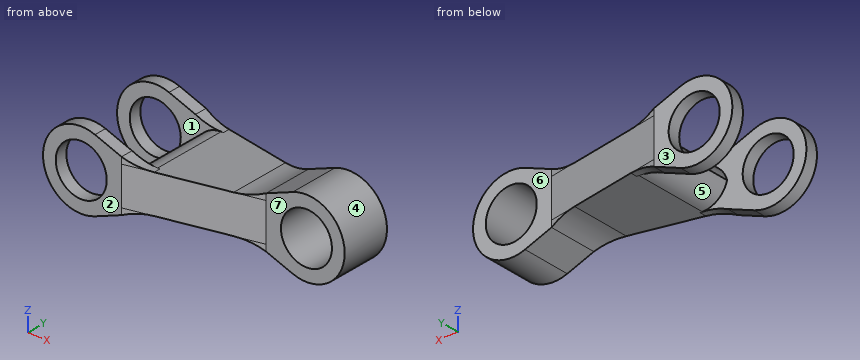
from build123d import *

# Parameters (mm, degrees)
SKETCH1_R           = 5.08
BOSS_EXTRUDE1_DEPTH = 10.16
SKETCH2_W           = 15.638324702
SKETCH2_H           = 15.24
CUT_EXTRUDE1_DEPTH  = 54.836616721
FILLET1_R           = 12.7
FILLET2_R           = 5.08


with BuildPart() as part:
    # Sketch1 → Boss-Extrude1 (new, symmetric)
    with BuildSketch(Plane(origin=(0, 0, 0), x_dir=(1, 0, 0), z_dir=(0, 1, 0))):
        with BuildLine():
            Line((2.735663722, 7.112), (8.018324702, 5.08))
            Line((8.018324702, 5.08), (8.018324702, 3.81))
            Line((8.018324702, 3.81), (32.621675298, 3.81))
            Line((32.621675298, 3.81), (32.621675298, 5.08))
            Line((32.621675298, 5.08), (37.904336278, 7.112))
            ThreePointArc((37.904336278, 7.112), (48.26, 0), (37.904336278, -7.112))
            Line((37.904336278, -7.112), (32.621675298, -5.08))
            Line((32.621675298, -5.08), (32.621675298, -3.81))
            Line((32.621675298, -3.81), (8.018324702, -3.81))
            Line((8.018324702, -3.81), (8.018324702, -5.08))
            Line((8.018324702, -5.08), (2.735663722, -7.112))
            ThreePointArc((2.735663722, -7.112), (-7.62, 0), (2.735663722, 7.112))
        make_face()
        with Locations(Location((0, 0, 0), (0, 0, 270))):
            Circle(SKETCH1_R, mode=Mode.SUBTRACT)
        with Locations(Location((40.64, 0, 0), (0, 0, 270))):
            Circle(SKETCH1_R, mode=Mode.SUBTRACT)
    extrude(amount=BOSS_EXTRUDE1_DEPTH, both=True)

    # Sketch2 → Cut-Extrude1 (cut, through all)
    with BuildSketch(Plane.XY.offset(13.97)):
        Polygon((8.018324702, 10.16), (32.621675298, 5.08), (48.26, 5.08), (48.26, 10.16), align=None)
        with Locations((0.199162351, 0)):
            Rectangle(SKETCH2_W, SKETCH2_H)
        Polygon((48.26, -10.16), (48.26, -5.08), (32.621675298, -5.08), (8.018324702, -10.16), align=None)
    extrude(amount=-CUT_EXTRUDE1_DEPTH, mode=Mode.SUBTRACT)

    # Fillet1
    # the kernel refuses this fillet: 12.7 mm, written as the material it adds along each edge
    with BuildSketch(Plane(origin=(32.621675298, 18.919504146, 3.81), x_dir=(-1, 0, 0), z_dir=(0, -1, 0))) as fillet1_piece_1_section:
        with BuildLine():
            CenterArc((5.535801658, -12.7), FILLET1_R, 90, 25.841932763)
            Line((0, -1.27), (0, 0))
            Line((0, 0), (5.535801658, 0))
        make_face()
    fillet1_piece_1 = extrude(amount=37.839008291, mode=Mode.PRIVATE)
    fillet1_piece_1 = split(fillet1_piece_1, bisect_by=Plane(origin=(37.374376864, -4.098681465, 3.81), z_dir=(-0.20221057606968723, 0.9793420663514691, 0)), keep=Keep.TOP, mode=Mode.PRIVATE)
    fillet1_piece_1 = split(fillet1_piece_1, bisect_by=Plane(origin=(29.880992297, 5.645885105, 3.81), z_dir=(-0.20221057606968723, -0.9793420663514691, 0)), keep=Keep.TOP, mode=Mode.PRIVATE)
    add(fillet1_piece_1)
    with BuildSketch(Plane(origin=(32.621675298, 18.919504146, -3.81), x_dir=(-1, 0, 0), z_dir=(0, -1, 0))) as fillet1_piece_2_section:
        with BuildLine():
            CenterArc((5.535801658, 12.7), FILLET1_R, 244.158067237, 25.841932763)
            Line((0, 1.27), (0, 0))
            Line((0, 0), (5.535801658, 0))
        make_face()
    fillet1_piece_2 = extrude(amount=37.839008291, mode=Mode.PRIVATE)
    fillet1_piece_2 = split(fillet1_piece_2, bisect_by=Plane(origin=(37.374376864, -4.098681465, -3.81), z_dir=(-0.20221057606968723, 0.9793420663514691, 0)), keep=Keep.TOP, mode=Mode.PRIVATE)
    fillet1_piece_2 = split(fillet1_piece_2, bisect_by=Plane(origin=(29.880992297, 5.645885105, -3.81), z_dir=(-0.20221057606968723, -0.9793420663514691, 0)), keep=Keep.TOP, mode=Mode.PRIVATE)
    add(fillet1_piece_2)
    with BuildSketch(Plane(origin=(8.018324702, -7.62, -3.81), x_dir=(1, 0, 0), z_dir=(0, -1, 0))) as fillet1_piece_3_section:
        with BuildLine():
            CenterArc((5.535801658, -12.7), FILLET1_R, 90, 25.841932763)
            Line((0, -1.27), (0, 0))
            Line((0, 0), (5.535801658, 0))
        make_face()
    fillet1_piece_3 = extrude(amount=16.379504146, mode=Mode.PRIVATE)
    fillet1_piece_3 = split(fillet1_piece_3, bisect_by=Plane(origin=(8.521329344, -10.056141643, -3.81), z_dir=(-0.20221057606968723, 0.9793420663514691, 0)), keep=Keep.TOP, mode=Mode.PRIVATE)
    add(fillet1_piece_3)
    with BuildSketch(Plane(origin=(8.018324702, 23.999504146, -3.81), x_dir=(1, 0, 0), z_dir=(0, -1, 0))) as fillet1_piece_4_section:
        with BuildLine():
            CenterArc((5.535801658, -12.7), FILLET1_R, 90, 25.841932763)
            Line((0, -1.27), (0, 0))
            Line((0, 0), (5.535801658, 0))
        make_face()
    fillet1_piece_4 = extrude(amount=16.379504146, mode=Mode.PRIVATE)
    fillet1_piece_4 = split(fillet1_piece_4, bisect_by=Plane(origin=(5.277641702, 10.725885105, -3.81), z_dir=(-0.20221057606968723, -0.9793420663514691, 0)), keep=Keep.TOP, mode=Mode.PRIVATE)
    add(fillet1_piece_4)
    with BuildSketch(Plane(origin=(8.018324702, -7.62, 3.81), x_dir=(0, 0, 1), z_dir=(0, -1, 0))) as fillet1_piece_5_section:
        with BuildLine():
            CenterArc((12.7, -5.535801658), FILLET1_R, 154.158067237, 25.841932763)
            Line((0, -5.535801658), (0, 0))
            Line((0, 0), (1.27, 0))
        make_face()
    fillet1_piece_5 = extrude(amount=16.379504146, mode=Mode.PRIVATE)
    fillet1_piece_5 = split(fillet1_piece_5, bisect_by=Plane(origin=(8.521329344, -10.056141643, 3.81), z_dir=(-0.20221057606968723, 0.9793420663514691, 0)), keep=Keep.TOP, mode=Mode.PRIVATE)
    add(fillet1_piece_5)
    with BuildSketch(Plane(origin=(8.018324702, 23.999504146, 3.81), x_dir=(0, 0, 1), z_dir=(0, -1, 0))) as fillet1_piece_6_section:
        with BuildLine():
            CenterArc((12.7, -5.535801658), FILLET1_R, 154.158067237, 25.841932763)
            Line((0, -5.535801658), (0, 0))
            Line((0, 0), (1.27, 0))
        make_face()
    fillet1_piece_6 = extrude(amount=16.379504146, mode=Mode.PRIVATE)
    fillet1_piece_6 = split(fillet1_piece_6, bisect_by=Plane(origin=(5.277641702, 10.725885105, 3.81), z_dir=(-0.20221057606968723, -0.9793420663514691, 0)), keep=Keep.TOP, mode=Mode.PRIVATE)
    add(fillet1_piece_6)

    # Fillet2
    # the kernel refuses this fillet: 5.08 mm, written as the material it takes off along each edge
    with BuildSketch(Plane(origin=(8.018324702, 7.62, -3.81), x_dir=(1, 0, 0), z_dir=(0, -1, 0)), Plane(origin=(8.018324702, 7.62, 3.81), x_dir=(0, 0, -1), z_dir=(0, -1, 0))) as fillet2_piece_1:
        with BuildLine():
            CenterArc((FILLET2_R, FILLET2_R), FILLET2_R, 180, 90)
            Line((0, FILLET2_R), (0, 0))
            Line((0, 0), (FILLET2_R, 0))
        make_face()
    extrude(amount=15.24, mode=Mode.SUBTRACT)


solid = part.part
Read the model definition and answer for the solid it produces. Units are mm, in the model's axes. Face numbers are marked on the shaded views. A direction names the side the tool comes from. Round coordinates to 2 decimals unless told otherwise and drop trailing zeros. Write each loop counter-clockwise with the first axis right and the second up, starting at its lowest first coordinate (ties: lowest second). Pieces come first, ordered by that corner, then holes. Notation, with made-up numbers: M -1.5,38.25 L 31.5,38.25 A24 ccw 31.5,51.25 Z; hole C -20,-7.5 d11. An arc over 180 degrees is marked long. Use a Markdown table: item, result.
1) For a pull along Y with two mould halves and no side action, classify the marked faces 1, 2, 3 and 4 as pulls with the +Y half, pulls with the -Y half, needs draft (parallel to the pull), parting line crosses it, or undercut.
Answers follow:
| item | result |
|---|---|
| face 1 | undercut |
| face 2 | pulls with the -Y half |
| face 3 | pulls with the +Y half |
| face 4 | needs draft |
2) The part is cut by section C-C (z = 1.75). Write down the section's boundary in (x, y), plus the area to 3 significant figures.
Answers follow:
| item | result |
|---|---|
| outline | M -7.42,-10.16 L -4.77,-10.16 L -4.77,-7.62 L -7.42,-7.62 Z; M -7.42,7.62 L -4.77,7.62 L -4.77,10.16 L -7.42,10.16 Z; M 4.77,-10.16 L 8.02,-10.16 L 32.62,-5.08 L 35.87,-5.08 L 35.87,5.08 L 32.62,5.08 L 8.02,10.16 L 4.77,10.16 L 4.77,7.62 L 9.01,7.62 L 9.01,-7.62 L 4.77,-7.62 Z; M 45.41,-5.08 L 48.06,-5.08 L 48.06,5.08 L 45.41,5.08 Z |
| area | 450 mm2 |
3) Flat-ended cylindrical pins translate along their axes: pin 1 (3 mm diameter, centred on y = -4, z = -4, fed in from -X); pin 2 (6 mm diameter, centred on x = 40.64, z = 0, fed in from +Y); pin 3 (7.5 mm diameter, centred on x = 40, z = 1.5, fed in from -Y); pin 4 (7 mm diameter, centred on x = 20, y = 0, fed in from +Z). Find the tip coordinate at first contact, or state that the pin passes through.
Answers follow:
| item | result |
|---|---|
| pin 1 | stops at x = 9.69 |
| pin 2 | passes through |
| pin 3 | stops at y = -5.08 |
| pin 4 | stops at z = 3.81 |
4) Straight lines are drawn through the part: line 1 along Z through (x, y) = (0, -9); line 2 along Y through (x, z) = (-2, 5.5); line 3 along X through (y, z) = (2, -2.25). For each, find the intervals that lie inside material, in ascending order. Write a range as [from, to].
Answers follow:
| item | result |
|---|---|
| line 1 | z = [-7.62, -5.08], [5.08, 7.62] |
| line 2 | y = [-10.16, -7.62], [7.62, 10.16] |
| line 3 | x = [9.44, 36.09], [45.19, 47.92] |
5) The part is cut by section A-A (y = 4.5). Write down the section's boundary in (x, z), plus the area to 3 significant figures.
Answers follow:
| item | result |
|---|---|
| outline | M 8.18,0 A5.08 ccw 13.1,-3.81 L 27.09,-3.81 A12.7 cw 32.62,-5.08 L 37.9,-7.11 A7.62 ccw long 37.9,7.11 L 32.62,5.08 A12.7 cw 27.09,3.81 L 13.1,3.81 A5.08 ccw Z; hole C 40.64,0 d10.16 |
| area | 296 mm2 |
6) The part is cut by section B-B (x = 40.64). Write down the section's boundary in (y, z).
Answers follow:
| item | result |
|---|---|
| outline | M -5.08,-7.62 L 5.08,-7.62 L 5.08,-5.08 L -5.08,-5.08 Z; M -5.08,5.08 L 5.08,5.08 L 5.08,7.62 L -5.08,7.62 Z |
7) The part is cut by section D-D (z = -6). Write down the section's boundary in (x, y).
Answers follow:
| item | result |
|---|---|
| outline | M -4.7,-10.16 L 5.63,-10.16 L 5.63,-7.62 L -4.7,-7.62 Z; M -4.7,7.62 L 5.63,7.62 L 5.63,10.16 L -4.7,10.16 Z; M 35.01,-5.08 L 45.34,-5.08 L 45.34,5.08 L 35.01,5.08 Z |
8) A tool of negligible diameter and unlimited length cuts with its end or side. For the marked faces 5, 6 and 7, from which of +Z, -Z, +X, -X, +Y, -Y can it reach the whole face along a straight path? Write none if from no direction.
Answers follow:
| item | result |
|---|---|
| face 5 | -Z, -X |
| face 6 | +Z, -Z, +X, +Y |
| face 7 | +Z, -Z, +X, -Y |
